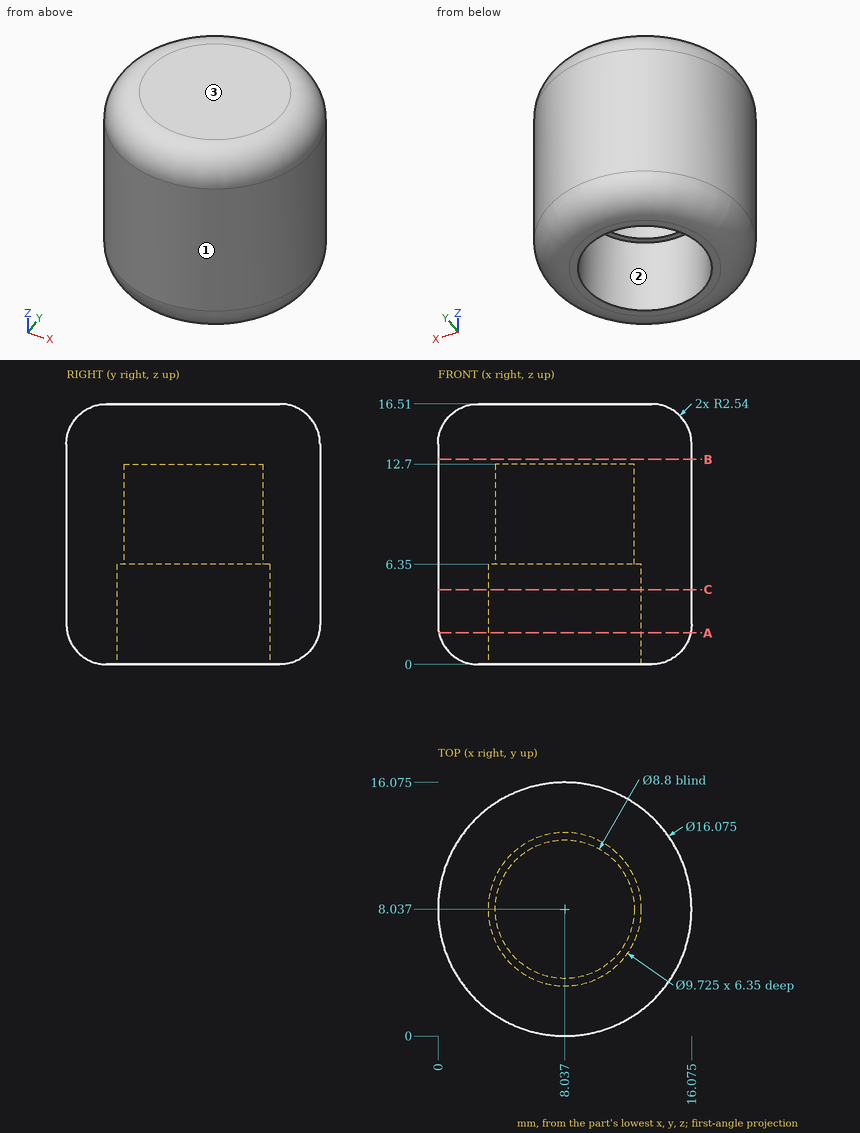
Verification items for this drawing (mm, ordinates from the low corner). Give positions to 0.01 mm unless a question says otherwise; leave off trailing zeros. Write each loop counter-clockwise with the first axis right and the second up, starting at its lowest first coordinate (ties: lowest second). Pieces come first, ordered by that corner, then holes.
1) Section check C-C, the plane z = 4.75. Record the boundary of the cut face in (x, y) (1 decimal).
2) Section check B-B, the plane z = 13. Record the boundary of the cut face in (x, y) (1 decimal).
3) Gauge pin test, flat ends, axial feed: pin 1 (4.5 mm diameter, centred on x = 7.5, y = 8, fed in from -Z); pin 2 (8 mm diameter, centred on x = 7.5, y = 7.5, fed in from -Z); pin 3 (1.5 mm diameter, centred on x = 4.5, z = 7.5, fed in from -Y). Record the tip position at first contact, or that the pin passes through.
4) Material ranges on L1, parallel to Z at x = 12, y = 10.25; L2, parallel to X at y = 7.5, z = 1.25 (1 decimal); L3, parallel to X at y = 10, z = 1 (1 decimal), recorded low to high.
5) Section check A-A, the plane z = 2. Record the boundary of the cut face in (x, y) (1 decimal).
6) Release check for a two-part mould opening along Y. For the marked faces 1, 2 and 3 record: pulls with the +Y half, pulls with the -Y half, needs draft (parallel to the pull), parting line crosses it, or undercut.
Computed:
1. outline: circle Ø16.1 at (8, 8); hole circle Ø9.7 at (8, 8)
2. outline: circle Ø16.1 at (8, 8)
3. pin 1: stops at z = 12.7
3. pin 2: stops at z = 6.35
3. pin 3: stops at y = 0.5
4. L1: z = 6.35 to 16.51
4. L2: x = 0.4 to 3.2, 12.9 to 15.7
4. L3: x = 0.8 to 3.6, 12.5 to 15.3
5. outline: circle Ø16 at (8, 8); hole circle Ø9.7 at (8, 8)
6. face 1: parting line crosses it
6. face 2: undercut
6. face 3: needs draft
